Geometry: see drawing. Coordinates: mm, zero at the bounding-box minimum. A direction names the side the tool comes from. Round coordinates to 2 decimals unless told otherwise and drop trailing zeros. Loops run counter-clockwise (first coordinate to the right, second up) from the corner with the lowest first, then second, coordinate; pieces in that order, holes last. Notation, with made-up numbers: (-27, -37) - (-23, -37) arc R20 ccw to (-23, -22) - close; hole circle Ø2 at (83, -23.75). An arc over 180 degrees is marked (long way). Answer in a Markdown table with one row per item. Add a question column.
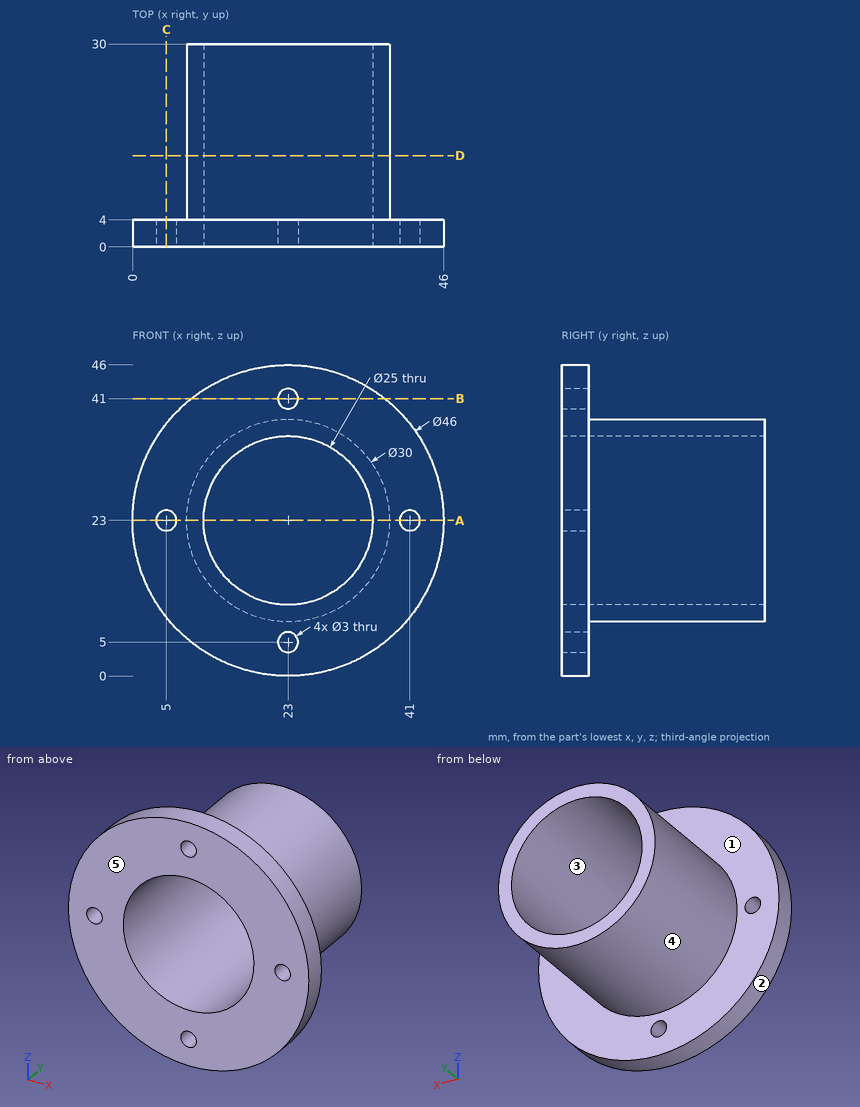
1) Section B-B, the plane z = 41. Return the cut outline in (x, y).
2) Contact query for flat-ended pins moving along their axis: pin 1 Ø3.5 at (x, z) = (41, 23) entering from +Y; pin 2 Ø5 at (x, y) = (23, 14) entering from -Z; pin 3 Ø8 at (x, y) = (7, 9) entering from -Z. Output: stop coordinate, or through.
3) Section A-A, the plane z = 23. Return the cut outline in (x, y).
4) Section C-C, the plane x = 5. Return the cut outline in (y, z).
5) Section D-D, the plane y = 13.5. Return the cut outline in (x, z).
6) Material intervals for line 1 along X through (y, z) = (7, 23); line 2 along Z through (x, y) = (23.5, 8.25); line 3 along Y through (x, z) = (7, 15), sorted ascending. Write a range as from..to.
7) Pull-direction query (Z, two-part tool) for the marked faces 1, 2 and 3; classes: pulls with the +Z half, pulls with the -Z half, needs draft (parallel to the pull), parting line crosses it, or undercut.
8) Reachability of the marked faces 4 and 5 from +Z, -Z, +X, -X, +Y, -Y: full face, straight path, thin tool, end or side. Return the list, or none.
Evaluation:
| question | item | result |
|---|---|---|
| 1 | outline | (8.68, 0) - (21.5, 0) - (21.5, 4) - (8.68, 4) - close; (24.5, 0) - (37.32, 0) - (37.32, 4) - (24.5, 4) - close |
| 2 | pin 1 | stops at y = 4 |
| 2 | pin 2 | stops at z = 8 |
| 2 | pin 3 | stops at z = 14 |
| 3 | outline | (0, 0) - (3.5, 0) - (3.5, 4) - (0, 4) - close; (6.5, 0) - (10.5, 0) - (10.5, 30) - (8, 30) - (8, 4) - (6.5, 4) - close; (35.5, 0) - (39.5, 0) - (39.5, 4) - (38, 4) - (38, 30) - (35.5, 30) - close; (42.5, 0) - (46, 0) - (46, 4) - (42.5, 4) - close |
| 4 | outline | (0, 8.68) - (4, 8.68) - (4, 21.5) - (0, 21.5) - close; (0, 24.5) - (4, 24.5) - (4, 37.32) - (0, 37.32) - close |
| 5 | outline | circle Ø30 at (23, 23); hole circle Ø25 at (23, 23) |
| 6 | line 1 | x = 8..10.5, 35.5..38 |
| 6 | line 2 | z = 8.01..10.51, 35.49..37.99 |
| 6 | line 3 | y = 0..4 |
| 7 | face 1 | needs draft |
| 7 | face 2 | parting line crosses it |
| 7 | face 3 | undercut |
| 8 | face 4 | +Y |
| 8 | face 5 | +Z, -Z, +X, -X, -Y |
